Can you work these out from the model? Positions are in its coordinate system, mm. A direction names the side the tool comes from. Coordinates: 2 decimals unless noted, no trailing zeros. Order: outer loops, then holes, each group sorted by start corner. A loop starts at its lowest first (then second) coordinate and runs counter-clockwise, first axis right, second up. Notation, with made-up numbers: (72.5, 8) -> (105.5, 8) arc R22 cw to (105.5, 43) -> close; hole circle Ø2 at (45, 25.5). An arc over 180 degrees is marked (long way). Answer in a Markdown table with one row per item. Add a question column.
1. On a 3-axis mill with a long thin cutter (end or side, diameter ignored), from which of +Z, -Z, +X, -X, +Y, -Y can I reach the whole of each face in a straight line? I mean faces 5 (the face through (5, -3, 20)), 6 (the face through (5, 0, 17)). Say none if no direction works.
2. Will this pin go through, and if not, where does the flat tip stop? pin 1 (1 mm diameter, centred on x = 9, z = 26.5, fed in from -Y).
3. Imagine slicing it at A-A on x = 10. Write out the boundary of the cut face in (y, z).
4. If I drill on line 1 along Z through (x, y) = (10, -6); line 2 along X through (y, z) = (-5.25, 11.25); line 3 along Z through (x, y) = (6.5, -6), over which ranges is the centre line in solid material (lowest first)? Write a range as [from, to].
5. We'd pull the mould along Z, two halves only. Please class faces 1 (the face through (10, -10, 0)), 2 (the face through (20, -10, 10)), 3 (the face through (10, -10, 30)), 4 (the face through (8.37, -10.14, 2.68)): pulls with the +Z half, pulls with the -Z half, needs draft (parallel to the pull), parting line crosses it, or undercut.
6. Imagine slicing it at D-D on x = 4. Write out the boundary of the cut face in (y, z).
7. Imagine slicing it at C-C on y = -10. Write out the boundary of the cut face in (x, z), plus the area to 3 significant figures.
8. Imagine slicing it at B-B on z = 10. Write out the boundary of the cut face in (x, y), plus the area to 3 significant figures.
from build123d import *

# Parameters (mm, degrees)
F0_W     = 20
F0_H     = 20
F1_DEPTH = 20
F2_R     = 7.5
F3_DEPTH = 10
F4_R     = 7.5
F5_DEPTH = 25


with BuildPart() as f1:
    # F0 (on Front) → F1 (new body)
    with BuildSketch(Plane.XZ):
        with Locations((10, 10)):
            Rectangle(F0_W, F0_H)
    extrude(amount=F1_DEPTH)

    # F2 (on face) → F3 (join)
    with BuildSketch(Plane.XY.offset(20)):
        with Locations((10, -10)):
            Circle(F2_R)
    extrude(amount=F3_DEPTH)

    # F4 (on face) → F5 (cut)
    with BuildSketch(Plane.XZ.offset(20)):
        with Locations((10, 10)):
            Circle(F4_R)
    extrude(amount=-F5_DEPTH, mode=Mode.SUBTRACT)


solid = f1.part
Answers follow:
| question | item | result |
|---|---|---|
| 1 | face 5 | +Z |
| 1 | face 6 | +Z, -Z, +X, -X, +Y |
| 2 | pin 1 | stops at y = -17.48 |
| 3 | outline | (-20, 0) -> (0, 0) -> (0, 2.5) -> (-20, 2.5) -> close; (-20, 17.5) -> (0, 17.5) -> (0, 20) -> (-2.5, 20) -> (-2.5, 30) -> (-17.5, 30) -> (-17.5, 20) -> (-20, 20) -> close |
| 4 | line 1 | z = [0, 2.5], [17.5, 30] |
| 4 | line 2 | x = [0, 2.6], [17.4, 20] |
| 4 | line 3 | z = [0, 3.37], [16.63, 30] |
| 5 | face 1 | pulls with the -Z half |
| 5 | face 2 | needs draft |
| 5 | face 3 | pulls with the +Z half |
| 5 | face 4 | undercut |
| 6 | outline | (-20, 0) -> (0, 0) -> (0, 5.5) -> (-20, 5.5) -> close; (-20, 14.5) -> (0, 14.5) -> (0, 20) -> (-5.5, 20) -> (-5.5, 30) -> (-14.5, 30) -> (-14.5, 20) -> (-20, 20) -> close |
| 7 | outline | (0, 0) -> (20, 0) -> (20, 20) -> (17.5, 20) -> (17.5, 30) -> (2.5, 30) -> (2.5, 20) -> (0, 20) -> close; hole circle Ø15 at (10, 10) |
| 7 | area | 373 mm² |
| 8 | outline | (0, -20) -> (2.5, -20) -> (2.5, 0) -> (0, 0) -> close; (17.5, -20) -> (20, -20) -> (20, 0) -> (17.5, 0) -> close |
| 8 | area | 100 mm² |
